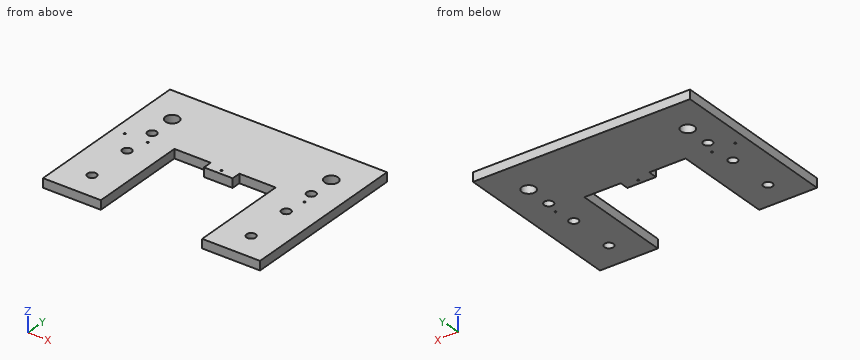
from build123d import *

# Parameters (mm, degrees)
SKETCH1_R           = 4.7371
SKETCH1_R_2         = 3.175
BOSS_EXTRUDE1_DEPTH = 6.35
SKETCH2_W           = 25.498289586
SKETCH2_H           = 6.35
CUT_EXTRUDE1_DEPTH  = 6.35
SKETCH3_R           = 0.635
CUT_EXTRUDE2_DEPTH  = 6.35


with BuildPart() as part:
    # Sketch1 → Boss-Extrude1 (new body)
    with BuildSketch(Plane.XY):
        Polygon((0, 0), (40.64, 0), (40.64, 63.5), (111.76, 63.5), (111.76, 0), (152.4, 0), (152.4, 69.85), (152.4, 120.65), (111.76, 120.65), (40.64, 120.65), (0, 120.65), (0, 69.85), align=None)
        with Locations((20.32, 95.25)):
            Circle(SKETCH1_R, mode=Mode.SUBTRACT)
        with Locations((132.08, 95.25)):
            Circle(SKETCH1_R, mode=Mode.SUBTRACT)
        with Locations((132.08, 76.2)):
            Circle(SKETCH1_R_2, mode=Mode.SUBTRACT)
        with Locations((20.32, 76.2)):
            Circle(SKETCH1_R_2, mode=Mode.SUBTRACT)
        with Locations((20.32, 52.3875)):
            Circle(SKETCH1_R_2, mode=Mode.SUBTRACT)
        with Locations((132.08, 52.3875)):
            Circle(SKETCH1_R_2, mode=Mode.SUBTRACT)
        with Locations((20.32, 19.05)):
            Circle(SKETCH1_R_2, mode=Mode.SUBTRACT)
        with Locations((132.08, 19.05)):
            Circle(SKETCH1_R_2, mode=Mode.SUBTRACT)
    extrude(amount=BOSS_EXTRUDE1_DEPTH)

    # Sketch2 → Cut-Extrude1 (cut)
    with BuildSketch(Plane(origin=(0, 0, 0), x_dir=(-1, 0, 0), z_dir=(0, 0, -1))):
        with Locations((-99.010855207, 66.675)):
            Rectangle(SKETCH2_W, SKETCH2_H)
        with Locations((-53.389144793, 66.675)):
            Rectangle(SKETCH2_W, SKETCH2_H)
    extrude(amount=-CUT_EXTRUDE1_DEPTH, mode=Mode.SUBTRACT)

    # Sketch3 → Cut-Extrude2 (cut)
    with BuildSketch(Plane(origin=(0, 0, 0), x_dir=(-1, 0, 0), z_dir=(0, 0, -1))):
        with Locations((-134.339930145, 66.675)):
            Circle(SKETCH3_R)
        with Locations((-98.219790435, 66.675)):
            Circle(SKETCH3_R)
        with Locations((-24.342185699, 66.675)):
            Circle(SKETCH3_R)
        with Locations((-76.2, 66.675)):
            Circle(SKETCH3_R)
        with Locations((-8.1140619, 66.675)):
            Circle(SKETCH3_R)
    extrude(amount=-CUT_EXTRUDE2_DEPTH, mode=Mode.SUBTRACT)


solid = part.part
Part model, mm, in its own coordinate system. Give positions to 0.01 mm unless a question says otherwise; leave off trailing zeros. Loops run counter-clockwise (first coordinate to the right, second up) from the corner with the lowest first, then second, coordinate; pieces in that order, holes last. Notation, with made-up numbers: (-39.5, -24) -> (0.5, -24) arc R25 ccw to (0.5, 10) -> close; hole circle Ø1 at (18, 62.5). An arc over 180 degrees is marked (long way). Write each question's results on one line, items separated by ' | '. Start each with the question number.
Q1. Wall check: L1, parallel to X at y = 65, z = 5.75; L2, parallel to X at y = 94, z = 2; L3, parallel to X at y = 29, z = 5. Give the ranges that are in metal, low to high.
Q2. Band-saw the part on C-C on x = 132.08. Count the separate pieces of the cut face and the enclosed holes in it, plus the area to 3 significant figures.
Q3. Pin check, flat tips, straight feed: P1, Ø3, axis at y = 33.5, z = 2.5, coming from the -X side; P2, Ø2, axis at x = 43, z = 4.5, coming from the -Y side; P3, Ø4, axis at x = 20.32, y = 76.2, coming from the -Z side; P4, Ø1.9, axis at x = 80, z = 2, coming from the -Y side. Stop position of each tip, or through.
Q4. Band-saw the part on B-B on y = 76.2. List the corners of the cut face in (x, z) (3 decimals).
Q5. Band-saw the part on A-A on y = 19.05. List the corners of the cut face in (x, z) (3 decimals), plus the area to 3 significant figures.
Results are:
1) L1: x = 0 to 40.64, 66.14 to 86.26, 111.76 to 152.4 | L2: x = 0 to 15.75, 24.89 to 127.51, 136.65 to 152.4 | L3: x = 0 to 40.64, 111.76 to 152.4
2) separate pieces: 5 | enclosed holes: 0 | area: 585 mm²
3) P1: stops at x = 0 | P2: stops at y = 69.85 | P3: passes through | P4: stops at y = 63.5
4) outline: (0, 0) -> (17.145, 0) -> (17.145, 6.35) -> (0, 6.35) -> close; (23.495, 0) -> (128.905, 0) -> (128.905, 6.35) -> (23.495, 6.35) -> close; (135.255, 0) -> (152.4, 0) -> (152.4, 6.35) -> (135.255, 6.35) -> close
5) outline: (0, 0) -> (17.145, 0) -> (17.145, 6.35) -> (0, 6.35) -> close; (23.495, 0) -> (40.64, 0) -> (40.64, 6.35) -> (23.495, 6.35) -> close; (111.76, 0) -> (128.905, 0) -> (128.905, 6.35) -> (111.76, 6.35) -> close; (135.255, 0) -> (152.4, 0) -> (152.4, 6.35) -> (135.255, 6.35) -> close | area: 435 mm²
